from build123d import *

# Parameters (mm, degrees)
SKETCH_R      = 2.25
PAD_DEPTH     = 2.8
SKETCH002_W   = 0.6
SKETCH002_H   = 0.6
PAD002_DEPTH  = 8
CHAMFER_SIZE  = 0.15
SKETCH003_R   = 0.15
PAD003_DEPTH  = 8
SKETCH004_R   = 2.225
SKETCH004_R_2 = 1.525
PAD004_DEPTH  = 7.2


with BuildPart() as part:
    # Sketch → Pad (new body)
    with BuildSketch(Plane.XY):
        Circle(SKETCH_R)
    extrude(amount=PAD_DEPTH)

    # Sketch002 → Pad002 (join)
    with BuildSketch(Plane(origin=(0, 0, 0), x_dir=(1, 0, 0), z_dir=(0, 0, -1))):
        Rectangle(SKETCH002_W, SKETCH002_H)
    extrude(amount=PAD002_DEPTH)

    # Chamfer
    chamfer_edges = [part.edges().sort_by_distance(p)[0] for p in [
        (0, -0.3, -8),
        (0.3, 0, -8),
        (0, 0.3, -8),
        (-0.3, 0, -8),
    ]]
    chamfer(chamfer_edges, length=CHAMFER_SIZE)

    # Sketch003 (on Face4 of Chamfer) → Pad003 (join)
    with BuildSketch(Plane(origin=(0, 0, 0), x_dir=(1, 0, 0), z_dir=(0, 0, -1))):
        with Locations((1.4, 0)):
            Circle(SKETCH003_R)
    extrude(amount=PAD003_DEPTH)

    # Sketch004 (on Face13 of Pad003) → Pad004 (join)
    with BuildSketch(Plane.XY.offset(2.8)):
        Circle(SKETCH004_R)
        Circle(SKETCH004_R_2, mode=Mode.SUBTRACT)
    extrude(amount=PAD004_DEPTH)


solid = part.part
Design review of the part built by this model. Coordinates are the model's own, in mm. A direction names the side the tool comes from. Round coordinates to 2 decimals unless told otherwise and drop trailing zeros. Loops run counter-clockwise (first coordinate to the right, second up) from the corner with the lowest first, then second, coordinate; pieces in that order, holes last. Notation, with made-up numbers: (41, -32) - (78, -32) arc R19 ccw to (78, -1) - close; hole circle Ø1 at (-10, -0.5). An arc over 180 degrees is marked (long way). One line per question, with ' | ' between items.
1. We need section A-A, the plane z = -2. State the section outline as (x, y) points.
Results are:
outline: (-0.3, -0.3) - (0.3, -0.3) - (0.3, 0.3) - (-0.3, 0.3) - close; circle Ø0.3 at (1.4, 0)
2. For L1, parallel to Y at x = 0, z = 6 (3 decimals); L2, parallel to X at y = 0, z = -3; L3, parallel to Z at x = -0.5, y = 1.35, list the stretches that pass through material, from the lowest coordinate up. Write a range as [from, to].
Results are:
L1: y = [-2.225, -1.525], [1.525, 2.225] | L2: x = [-0.3, 0.3], [1.25, 1.55] | L3: z = [0, 2.8]
3. We need section B-B, the plane z = 4. State the section outline as (x, y) points (3 decimals), and give its area (3 significant figures).
Results are:
outline: circle Ø4.45 at (0, 0); hole circle Ø3.05 at (0, 0) | area: 8.25 mm²
4. Draft analysis for pull direction X (two halves, no side actions). For faces 1 (the face through (0, 2, 10)), 2 (the face through (-1.524, 0.067, 6.35)), 3 (the face through (-0.482, -2.172, 6.35)), state which applies: released by +X, released by -X, zero draft, split by the parting line, or undercut.
Results are:
face 1: zero draft | face 2: undercut | face 3: split by the parting line
5. Clearance check with flat-ended pins moving along their axes: P1, Ø0.5, axis at y = 0, z = -2.5, coming from the -X side; P2, Ø1.3, axis at x = -0.5, y = 0.5, coming from the +Z side. State where each tip first meets the part, or that it passes through.
Results are:
P1: stops at x = -0.3 | P2: stops at z = 2.8
6. For faces 4 (the face through (-0.29, 2.23, 1.38)), 5 (the face through (0, 0, 2.8)), list the 3-axis set-ups (+Z, -Z, +X, -X, +Y, -Y) from which the entire face can be reached by the end or side of a thin tool; tool diameter is ignored.
Results are:
face 4: +Z, -Z | face 5: +Z
